Read the model definition and answer for the solid it produces. Units are mm, in the model's axes. A direction names the side the tool comes from. Coordinates: 2 decimals unless noted, no trailing zeros. Order: outer loops, then holes, each group sorted by start corner. A loop starts at its lowest first (then second) coordinate and runs counter-clockwise, first axis right, second up. Notation, with made-up numbers: M 75.25,23.5 L 106.25,23.5 A16 ccw 106.25,33.5 Z; hole C -30.5,43 d3. An arc over 180 degrees is marked long. One line per question, with ' | ' between items. Start each with the question number.
1) The mould has two halves that part along X. Classify faces 1 (the face through (0, 0, 145)), 2 (the face through (0, -13, -33)), 3 (the face through (-17.5, 0, 50)): +X half, -X half, draft (parallel to the pull), parting line (faces both ways), or undercut.
2) Find section A-A, the plane y = 7. Write down the section's boundary in (x, z), plus the area to 3 significant figures.
3) Consider probe 1 along X at (y, z) = (2.5, 82); probe 2 along Z at (x, y) = (10, 8.5); probe 3 along Z at (x, y) = (-7.5, 13). Determine where each line is inside the solid, lowest interval first.
4) A tool of negligible diameter and unlimited length cuts with its end or side. For faces 4 (the face through (15.5, 9, 62)), 5 (the face through (0, 0, -48)), from which of +Z, -Z, +X, -X, +Y, -Y can it reach the whole face along a straight path? Write none if from no direction.
5) Find section B-B, the plane z = 6. Write down the section's boundary in (x, y).
from build123d import *

# Parameters (mm, degrees)
BOSS_EXTRUDE3_DEPTH = 125
SKETCH4_W           = 35
SKETCH4_H           = 35
BOSS_EXTRUDE4_DEPTH = 20
CUT_EXTRUDE2_DEPTH  = 17
SKETCH6_W           = 35
SKETCH6_H           = 35
BOSS_EXTRUDE5_DEPTH = 48
CUT_EXTRUDE3_START  = -20
CUT_EXTRUDE3_DEPTH  = 20
CUT_EXTRUDE4_DEPTH  = 26
FILLET1_R           = 12.7
FILLET2_R           = 2


with BuildPart() as part:
    # Sketch1 → Boss-Extrude3 (new body)
    with BuildSketch(Plane.XY):
        with BuildLine():
            Line((0, -17.5), (-17.5, -17.5))
            Line((-17.5, -17.5), (-17.5, 0))
            Line((-17.5, 0), (-17.5, 17.5))
            Line((-17.5, 17.5), (-15.5, 17.5))
            Line((-15.5, 17.5), (-15.5, 0))
            ThreePointArc((-15.5, 0), (0, -15.5), (15.5, 0))
            Line((15.5, 0), (15.5, 17.5))
            Line((15.5, 17.5), (17.5, 17.5))
            Line((17.5, 17.5), (17.5, 0))
            Line((17.5, 0), (17.5, -17.5))
            Line((17.5, -17.5), (0, -17.5))
        make_face()
    extrude(amount=BOSS_EXTRUDE3_DEPTH)

    # Sketch4 → Boss-Extrude4 (add)
    with BuildSketch(Plane.XY.offset(125)):
        Rectangle(SKETCH4_W, SKETCH4_H)
    extrude(amount=BOSS_EXTRUDE4_DEPTH)

    # Sketch5 → Cut-Extrude2 (cut)
    with BuildSketch(Plane(origin=(0, 0, 125), x_dir=(-1, 0, 0), z_dir=(0, 0, -1))):
        with BuildLine():
            Line((-5, 0), (-5, 17.5))
            Line((-5, 17.5), (5, 17.5))
            Line((5, 17.5), (5, 0))
            ThreePointArc((5, 0), (0, -5), (-5, 0))
        make_face()
    extrude(amount=-CUT_EXTRUDE2_DEPTH, mode=Mode.SUBTRACT)

    # Sketch6 → Boss-Extrude5 (add)
    with BuildSketch(Plane(origin=(0, 0, 0), x_dir=(-1, 0, 0), z_dir=(0, 0, -1))):
        Rectangle(SKETCH6_W, SKETCH6_H)
    extrude(amount=BOSS_EXTRUDE5_DEPTH)

    # Sketch7 → Cut-Extrude3 (cut)
    with BuildSketch(Plane.XY.offset(CUT_EXTRUDE3_START)):
        with BuildLine():
            Line((-5, 0), (-5, 17.5))
            Line((-5, 17.5), (5, 17.5))
            Line((5, 17.5), (5, 0))
            ThreePointArc((5, 0), (0, -5), (-5, 0))
        make_face()
    extrude(amount=CUT_EXTRUDE3_DEPTH, mode=Mode.SUBTRACT)

    # Sketch8 → Cut-Extrude4 (cut)
    with BuildSketch(Plane.XY.offset(-20)):
        with BuildLine():
            Line((-13, 0), (-13, 27.339362416))
            Line((-13, 27.339362416), (13, 27.339362416))
            Line((13, 27.339362416), (13, 0))
            ThreePointArc((13, 0), (0, -13), (-13, 0))
        make_face()
    extrude(amount=-CUT_EXTRUDE4_DEPTH, mode=Mode.SUBTRACT)

    # Fillet1
    # the kernel refuses this fillet: 12.7 mm, written as the material it adds along each edge
    with BuildSketch(Plane(origin=(13, 17.5, -20), x_dir=(-1, 0, 0), z_dir=(0, -1, 0)), Plane(origin=(-13, 0, -20), x_dir=(1, 0, 0), z_dir=(0, 1, 0))) as fillet1_piece_1:
        with BuildLine():
            CenterArc((12.7, 11.798304963), FILLET1_R, 180, 68.279526527)
            Line((0, 11.798304963), (-0.254, 11.798304963))
            Line((-0.254, 11.798304963), (-0.254, 0))
            Line((-0.254, 0), (0, -0.254))
            ThreePointArc((0, -0.254), (4, -0.254), (7.906, -0.235966099))
            Line((7.906, -0.235966099), (8, 0))
        make_face()
    extrude(amount=17.5)
    with BuildSketch(Plane(origin=(0, 0, -20), x_dir=(1, 0, 0), z_dir=(0, 1, 0))) as fillet1_piece_2:
        with BuildLine():
            CenterArc((0.3, 11.798304963), FILLET1_R, 291.720473473, 68.279526527)
            Line((13, 11.798304963), (13.254, 11.798304963))
            Line((13.254, 11.798304963), (13.254, 0))
            Line((13.254, 0), (13, -0.254))
            ThreePointArc((13, -0.254), (9, -0.254), (5.094, -0.235966099))
            Line((5.094, -0.235966099), (5, 0))
        make_face()
    revolve(axis=Axis((0, 0, -20), (0, 0, -1)), revolution_arc=180)
    with BuildSketch(Plane(origin=(13, 17.5, -46), x_dir=(0, 0, 1), z_dir=(0, -1, 0))) as fillet1_piece_3:
        with BuildLine():
            CenterArc((FILLET1_R, FILLET1_R), FILLET1_R, 180, 90)
            Line((0, FILLET1_R), (-FILLET1_R * 0.02, FILLET1_R))
            Line((-FILLET1_R * 0.02, FILLET1_R), (-FILLET1_R * 0.02, -FILLET1_R * 0.02))
            Line((-FILLET1_R * 0.02, -FILLET1_R * 0.02), (FILLET1_R, -FILLET1_R * 0.02))
            Line((FILLET1_R, -FILLET1_R * 0.02), (FILLET1_R, 0))
        make_face()
    extrude(amount=17.5)
    with BuildSketch(Plane(origin=(0, 0, -46), x_dir=(1, 0, 0), z_dir=(0, 1, 0))) as fillet1_piece_4:
        with BuildLine():
            CenterArc((13 - FILLET1_R, -FILLET1_R), FILLET1_R, 0, 90)
            Line((13, -FILLET1_R), (13 + FILLET1_R * 0.02, -FILLET1_R))
            Line((13 + FILLET1_R * 0.02, -FILLET1_R), (13 + FILLET1_R * 0.02, FILLET1_R * 0.02))
            Line((13 + FILLET1_R * 0.02, FILLET1_R * 0.02), (13 - FILLET1_R, FILLET1_R * 0.02))
            Line((13 - FILLET1_R, FILLET1_R * 0.02), (13 - FILLET1_R, 0))
        make_face()
    revolve(axis=Axis((0, 0, -46), (0, 0, -1)), revolution_arc=180)
    with BuildSketch(Plane(origin=(-13, 0, -46), x_dir=(1, 0, 0), z_dir=(0, 1, 0))) as fillet1_piece_5:
        with BuildLine():
            CenterArc((FILLET1_R, -FILLET1_R), FILLET1_R, 90, 90)
            Line((0, -FILLET1_R), (-FILLET1_R * 0.02, -FILLET1_R))
            Line((-FILLET1_R * 0.02, -FILLET1_R), (-FILLET1_R * 0.02, FILLET1_R * 0.02))
            Line((-FILLET1_R * 0.02, FILLET1_R * 0.02), (FILLET1_R, FILLET1_R * 0.02))
            Line((FILLET1_R, FILLET1_R * 0.02), (FILLET1_R, 0))
        make_face()
    extrude(amount=17.5)

    # Fillet2
    fillet2_edges = [part.edges().sort_by_distance(p)[0] for p in [
        (0, -5, -20),
        (-5, 8.75, -20),
        (5, 8.75, -20),
        (0, -5, 0),
        (5, 8.75, 0),
        (-5, 8.75, 0),
    ]]
    fillet(fillet2_edges, radius=FILLET2_R)


solid = part.part
Report:
1) face 1: draft | face 2: undercut | face 3: -X half
2) outline: M -17.5,-48 L 17.5,-48 L 17.5,145 L -17.5,145 Z; hole M -15.5,0 L -7,0 A2 cw -5,-2 L -5,-18.71 A2 cw -6.09,-20.49 A12.7 ccw -13,-31.8 L -13,-33.3 A12.7 ccw -0.3,-46 L 0.3,-46 A12.7 ccw 13,-33.3 L 13,-31.8 A12.7 ccw 6.09,-20.49 A2 cw 5,-18.71 L 5,-2 A2 cw 7,0 L 15.5,0 L 15.5,125 L 5,125 L 5,142 L -5,142 L -5,125 L -15.5,125 Z | area: 1,950 mm^2
3) probe 1: x = -17.5 to -15.5, 15.5 to 17.5 | probe 2: z = -48 to -41.5, -23.6 to 0, 125 to 145 | probe 3: z = -48 to -43.76, -21.34 to 0, 125 to 145
4) face 4: +Y | face 5: -Z, +X, -X, +Y, -Y
5) outline: M -17.5,-17.5 L 17.5,-17.5 L 17.5,17.5 L 15.5,17.5 L 15.5,0 A15.5 cw -15.5,0 L -15.5,17.5 L -17.5,17.5 Z
